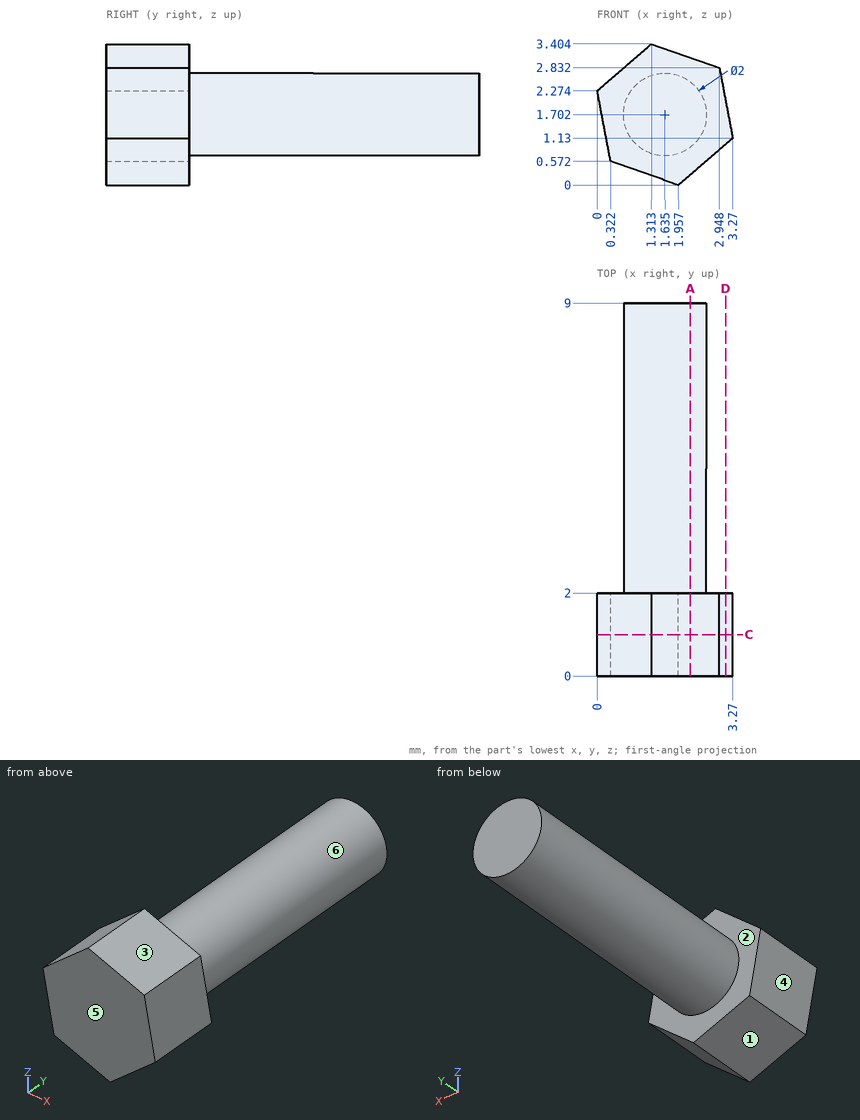
Job drawing, mm, ordinate dimensions from the low corner. One solid piece. A direction names the side the tool comes from. Coordinates: 2 decimals unless noted, no trailing zeros. Loops run counter-clockwise (first coordinate to the right, second up) from the corner with the lowest first, then second, coordinate; pieces in that order, holes last. Notation, with made-up numbers: (10, 32) - (30, 32) arc R16 ccw to (30, 44) - close; hole circle Ø4 at (80, 81.25). An arc over 180 degrees is marked (long way). Answer as a JSON object with one key per item and string values. Group by question number.
(1) Probe line 1 along Y through (x, z) = (0.45, 1.3); line 2 along Z through (x, y) = (2.05, 1) (1 decimal); line 3 along X through (y, z) = (3.5, 2). List the from-to ranges inside material, lowest first.
(2) Tool access for the marked faces 1 and 2: list every direction of +Z, -Z, +X, -X, +Y, -Y with a clear straight run to the whole face (end or side of a thin tool).
(3) Flat gauge pin, fed straight in: pin 1 (1 mm diameter, centred on y = 8, z = 1, fed in from -X) (1 decimal). Where does the tip first touch, or does it go through?
(4) Cut at D-D (x = 3.1). Give the cut face in (y, z).
(5) Two-plate mould, pull along X, no slides. Class the marked faces 3, 4, 5 and 6: released by +X, released by -X, zero draft, split by the parting line, or undercut.
(6) Cut at A-A (x = 2.25). Give the cut face in (y, z) (1 decimal), then the cut area to 3 significant figures.
(7) Cut at C-C (y = 1). Give the cut face in (x, z).
Geometry says:
{
 "1": {"line 1": "y = 0 to 2", "line 2": "z = 0.1 to 3.1", "line 3": "x = 0.68 to 2.59"},
 "2": {"face 1": "-Z, -X, +Y, -Y", "face 2": "+Y"},
 "3": {"pin 1": "stops at x = 0.7"},
 "4": {"outline": "(0, 0.98) - (2, 0.98) - (2, 2.03) - (0, 2.03) - close"},
 "5": {"face 3": "released by +X", "face 4": "released by -X", "face 5": "zero draft", "face 6": "split by the parting line"},
 "6": {"outline": "(0, 0.3) - (2, 0.3) - (2, 0.9) - (9, 0.9) - (9, 2.5) - (2, 2.5) - (2, 3.1) - (0, 3.1) - close", "area": "16.7 mm^2"},
 "7": {"outline": "(0, 2.27) - (0.32, 0.57) - (1.96, 0) - (3.27, 1.13) - (2.95, 2.83) - (1.31, 3.4) - close"}
}
